Here's how the part is built. I have some questions about the finished solid (model axes, mm). A direction names the side the tool comes from. Give positions to 0.01 mm unless a question says otherwise; leave off trailing zeros. Write each loop counter-clockwise with the first axis right and the second up, starting at its lowest first coordinate (ties: lowest second). Pieces come first, ordered by that corner, then holes. Notation, with made-up numbers: M 10,53 L 33,53 A8 ccw 33,57 Z; hole C 36.25,5.25 d8. An arc over 180 degrees is marked long. Answer as CSV lines item,"result". Start each with the question number.
Q1. Suppose I cut it at B-B (x = -6.35). Write out the boundary of the cut face in (y, z).
Q2. Suppose I cut it at A-A (y = -12). Write out the boundary of the cut face in (x, z).
Q3. Thinking about a two-plate mould opening in X: for faces 4 (the flat face through (0, 8, 3.5)), 5 (the cylindrical face through (-5.085, -11.466, 5.544)), 6 (the flat face through (12.7, 0, 0)), which applies, +X half, -X half, draft (parallel to the pull), parting line (faces both ways), or undercut?
Q4. On a 3-axis mill with a long thin cutter (end or side, diameter ignored), from which of +Z, -Z, +X, -X, +Y, -Y can I reach the whole of each face in a straight line? I mean faces 1 (the flat face through (0, 8, -3.5)), 2 (the flat face through (6, -8.89, -6)), 3 (the flat face through (0, -13.97, 0)). Say none if no direction works.
Q5. Suppose I cut it at C-C (z = 1.5). Write out the boundary of the cut face in (x, y).
Q6. If I drill on line 1 along X through (y, z) = (-12.45, 6.35); line 2 along Y through (x, z) = (-0.5, 0); line 3 along X through (y, z) = (-10.5, 5.25), over which ranges is the centre line in solid material (lowest first)?
Q7. For pin 1 (1.5 mm diameter, centred on x = -6, z = 6.5, fed in from -Y); pin 2 (3.5 mm diameter, centred on x = 6.35, z = 6.35, fed in from -Y), each with a flat end and sliding along its axis, tell me the tip position at first contact or that it passes through.
Q8. Suppose I cut it at D-D (y = 8.5). Write out the boundary of the cut face in (x, z), then the cut area to 3 significant figures.
```python
from build123d import *

# Parameters (mm, degrees)
SKETCH1_W           = 25.4
SKETCH1_H           = 25.4
BOSS_EXTRUDE1_DEPTH = 13.97
SKETCH2_R           = 1.5
CUT_EXTRUDE1_DEPTH  = 5.08
SKETCH3_W           = 7
SKETCH3_H           = 3
CUT_EXTRUDE2_DEPTH  = 32.648236918
FILLET1_R           = 1


with BuildPart() as part:
    # Sketch1 → Boss-Extrude1 (new, symmetric)
    with BuildSketch(Plane(origin=(0, 0, 0), x_dir=(1, 0, 0), z_dir=(0, 1, 0))):
        Rectangle(SKETCH1_W, SKETCH1_H)
    extrude(amount=BOSS_EXTRUDE1_DEPTH, both=True)

    # Sketch2 → Cut-Extrude1 (cut)
    with BuildSketch(Plane.XZ.offset(13.97)):
        with Locations(Location((-6.35, 6.35, 0), (0, 0, 270))):
            Circle(SKETCH2_R)
        with Locations(Location((6.35, 6.35, 0), (0, 0, 270))):
            Circle(SKETCH2_R)
        with Locations(Location((6.35, -6.35, 0), (0, 0, 270))):
            Circle(SKETCH2_R)
        with Locations(Location((-6.35, -6.35, 0), (0, 0, 270))):
            Circle(SKETCH2_R)
    extrude(amount=-CUT_EXTRUDE1_DEPTH, mode=Mode.SUBTRACT)

    # Sketch3 → Cut-Extrude2 (cut, through all)
    with BuildSketch(Plane(origin=(12.7, 0, 0), x_dir=(0, 0, -1), z_dir=(1, 0, 0))):
        with Locations((0, 8.03)):
            Rectangle(SKETCH3_W, SKETCH3_H)
    extrude(amount=-CUT_EXTRUDE2_DEPTH, mode=Mode.SUBTRACT)

    # Fillet1
    fillet1_edges = [part.edges().sort_by_distance(p)[0] for p in [
        (-12.7, 13.97, 0),
        (0, 13.97, 12.7),
        (12.7, 13.97, 0),
        (12.7, 0, 12.7),
        (-12.7, 0, 12.7),
        (-12.7, 0, -12.7),
        (12.7, 0, -12.7),
        (0, 13.97, -12.7),
    ]]
    fillet(fillet1_edges, radius=FILLET1_R)


solid = part.part
```
Resolved:
1,outline,"M -13.97,-12.7 L 12.97,-12.7 A1 ccw 13.97,-11.7 L 13.97,11.7 A1 ccw 12.97,12.7 L -13.97,12.7 L -13.97,7.85 L -8.89,7.85 L -8.89,4.85 L -13.97,4.85 L -13.97,-4.85 L -8.89,-4.85 L -8.89,-7.85 L -13.97,-7.85 Z; hole M 6.53,-3.5 L 9.53,-3.5 L 9.53,3.5 L 6.53,3.5 Z"
2,outline,"M -12.7,-11.7 A1 ccw -11.7,-12.7 L 11.7,-12.7 A1 ccw 12.7,-11.7 L 12.7,11.7 A1 ccw 11.7,12.7 L -11.7,12.7 A1 ccw -12.7,11.7 Z; hole C -6.35,-6.35 d3; hole C -6.35,6.35 d3; hole C 6.35,-6.35 d3; hole C 6.35,6.35 d3"
3,face 4,"draft"
3,face 5,"undercut"
3,face 6,"+X half"
4,face 1,"+X, -X"
4,face 2,"-Y"
4,face 3,"+Z, -Z, +X, -X, -Y"
5,outline,"M -12.7,-13.97 L 12.7,-13.97 L 12.7,6.53 L -12.7,6.53 Z; M -12.7,9.53 L 12.7,9.53 L 12.7,12.97 A1 ccw 11.7,13.97 L -11.7,13.97 A1 ccw -12.7,12.97 Z"
6,line 1,"-12.7 to -7.85, -4.85 to 4.85, 7.85 to 12.7"
6,line 2,"-13.97 to 6.53, 9.53 to 13.97"
6,line 3,"-12.7 to -7.37, -5.33 to 5.33, 7.37 to 12.7"
7,pin 1,"y = -8.89"
7,pin 2,"y = -13.97"
8,outline,"M -12.7,-11.7 A1 ccw -11.7,-12.7 L 11.7,-12.7 A1 ccw 12.7,-11.7 L 12.7,-3.5 L -12.7,-3.5 Z; M -12.7,3.5 L 12.7,3.5 L 12.7,11.7 A1 ccw 11.7,12.7 L -11.7,12.7 A1 ccw -12.7,11.7 Z"
8,area,"467 mm^2"
